```python
from build123d import *

# Parameters (mm, degrees)
BOSS_EXTRUDE1_DEPTH = 10


with BuildPart() as part:
    # Sketch1 → Boss-Extrude1 (new body)
    with BuildSketch(Plane.XY):
        with BuildLine():
            Line((0, 0), (0, 205))
            Line((0, 205), (10, 215))
            Line((10, 215), (122, 215))
            Line((122, 215), (122, 151))
            Line((122, 151), (112, 141))
            Line((112, 141), (44, 141))
            ThreePointArc((44, 141), (41.171572875, 139.828427125), (40, 137))
            Line((40, 137), (40, 0))
            Line((40, 0), (0, 0))
        make_face()
    extrude(amount=BOSS_EXTRUDE1_DEPTH)


solid = part.part
```
The model under review builds one solid part; all positions refer to its coordinate system, in mm. A direction names the side the tool comes from. Round coordinates to 2 decimals unless told otherwise and drop trailing zeros. Loops run counter-clockwise (first coordinate to the right, second up) from the corner with the lowest first, then second, coordinate; pieces in that order, holes last. Notation, with made-up numbers: (-29, -3) -> (-15, -3) arc R26 ccw to (-15, 34) -> close; hole circle Ø10 at (42.5, 71.25). An arc over 180 degrees is marked (long way). Answer as a JSON object with one key per item and string values. Group by question number.
1) We need section B-B on y = 68. Write out the cut boundary in (x, z).
2) For faces 1 (the face through (0, 101, 5)), 2 (the face through (40, 69, 5)), list the 3-axis set-ups (+Z, -Z, +X, -X, +Y, -Y) from which the entire face can be reached by the end or side of a thin tool; tool diameter is ignored.
3) For pin 1 Ø3 at (y, z) = (40, 3) entering from +X; pin 2 Ø3 at (x, z) = (67, 3) entering from -Y, all flat-tipped, find the tip position at first contact; note any pin that passes through.
4) For line 1 (X direction, y = 107, z = 7.25); line 2 (Y direction, x = 82.5, z = 1); line 3 (Y direction, x = 43, z = 7.5), list the stretches that pass through material, from the lowest coordinate up. Write a range as [from, to].
5) We need section A-A on z = 2. Write out the cut boundary in (x, y), then the cut area to 3 significant figures.
6) We need section C-C on x = 101.5. Write out the cut boundary in (y, z), then the cut area to 3 significant figures.
Result set:
{
 "1": {"outline": "(0, 0) -> (40, 0) -> (40, 10) -> (0, 10) -> close"},
 "2": {"face 1": "+Z, -Z, -X, +Y, -Y", "face 2": "+Z, -Z, +X, -Y"},
 "3": {"pin 1": "x = 40", "pin 2": "y = 141"},
 "4": {"line 1": "[0, 40]", "line 2": "[141, 215]", "line 3": "[140.87, 215]"},
 "5": {"outline": "(0, 0) -> (40, 0) -> (40, 137) arc R4 cw to (44, 141) -> (112, 141) -> (122, 151) -> (122, 215) -> (10, 215) -> (0, 205) -> close", "area": "14,600 mm²"},
 "6": {"outline": "(141, 0) -> (215, 0) -> (215, 10) -> (141, 10) -> close", "area": "740 mm²"}
}
